Autodesk Inventor part; units mm, degrees
ref_plane "YZ Plane" through (0, 0, 0) normal (1, 0, 0) x (0, 1, 0)
ref_plane "XZ Plane" through (0, 0, 0) normal (0, 1, 0) x (-1, 0, 0)
ref_plane "XY Plane" through (0, 0, 0) normal (0, 0, 1) x (1, 0, 0)
sketch "Sketch1" plane through (0, 0, 0) normal (0, 1, 0) x (-1, 0, 0)
  line L0 (4.9, 2.9) -> (-4.9, 2.9)
  line L1 (-4.9, 2.9) -> (-4.9, -2.9)
  line L2 (-4.9, -2.9) -> (4.9, -2.9)
  line L3 (4.9, -2.9) -> (4.9, 2.9)
  point P0 (0, 0)
  dimension "d0" = 9.8
  dimension "d1" = 5.8
  dimension "d2" = 2.9
  dimension "d3" = 4.9
extrude "Extrusion1" add sketch "Sketch1" along normal blind 20
sketch "Sketch2" plane through (0, 0, 0) normal (0, -1, 0) x (1, 0, 0)
  circle A0 centre (0, 0) radius 10
  dimension "d6" = 20
extrude "Extrusion2" add sketch "Sketch2" along normal blind 3
sketch "Sketch3" plane through (0, 20, 0) normal (0, 1, 0) x (1, 0, 0)
  line L0 (-4.9, 2.9) -> (-4.9, -2.9)
  line L1 (-4.9, -2.9) -> (4.9, -2.9)
  line L2 (-4.9, 2.9) -> (4.9, 2.9)
  line L3 (4.9, 2.9) -> (4.9, -2.9)
  line L4 (4.9, -2.9) -> (-4.9, -2.9)
  line L5 (-4.9, -2.9) -> (-4.9, 2.9)
  point P0 (0, 0)
extrude "Extrusion3" cut sketch "Sketch3" against normal up to surface (20 mm away)
sketch "Sketch4" plane through (0, 0, 0) normal (1, 0, 0) x (0, 1, 0)
  circle A0 centre (9, 0) radius 10
  line L0 (-3, 10) -> (-3, -10)
  point P0 (0, 0)
  point P1 (-3, 0)
  dimension "d11" = 20
  dimension "d12" = 12
  dimension "d13" = 0
extrude "Extrusion4" cut sketch "Sketch4" along normal through all both and the other way through all
sketch "Sketch5" plane through (0, -3, 0) normal (0, -1, 0) x (1, 0, 0)
  line L0 (-4.8, 2.8) -> (4.8, 2.8)
  line L1 (4.8, 2.8) -> (4.8, -2.8)
  line L2 (4.8, -2.8) -> (-4.8, -2.8)
  line L3 (-4.8, -2.8) -> (-4.8, 2.8)
  point P0 (0, 0)
  dimension "d16" = 9.6
  dimension "d17" = 5.6
  dimension "d18" = 2.8
  dimension "d19" = 4.8
extrude "Extrusion5" add sketch "Sketch5" against normal blind 23
sketch "Sketch6" plane through (0, -3, 0) normal (0, -1, 0) x (1, 0, 0)
  line L0 (8, 10) -> (10, 10)
  line L1 (10, 10) -> (10, -10)
  line L2 (10, -10) -> (8, -10)
  line L3 (8, -10) -> (8, 10)
  line L4 (-10, 10) -> (-8, 10)
  line L5 (-8, 10) -> (-8, -10)
  line L6 (-8, -10) -> (-10, -10)
  line L7 (-10, -10) -> (-10, 10)
  circle A0 centre (0, 0) radius 10
  point P0 (-9, -10)
  point P1 (-9, 10)
  dimension "d22" = 20
  dimension "d23" = 10
  dimension "d24" = 2
  dimension "d25" = 10
  dimension "d26" = 8
  dimension "d27" = 2
  dimension "d28" = 0
  dimension "d29" = 0
extrude "Extrusion6" cut sketch "Sketch6" against normal through all contours L0 L1 A0 L3 | A0 L3 | L1 L2 L3 A0 | A0 L7 L4 L5 | L5 A0 | L5 L6 L7 A0
properties part number "Pin"
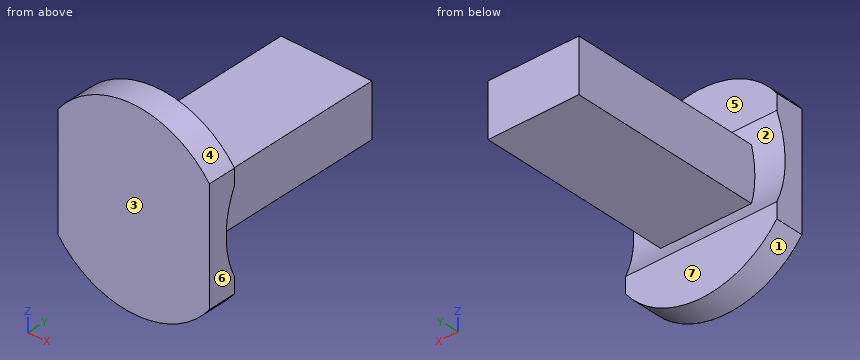
Geometry: final body of the model. Coordinates: model frame, mm. Face numbers are marked on the shaded views. A direction names the side the tool comes from. Give positions to 0.01 mm unless a question says otherwise; leave off trailing zeros. Loops run counter-clockwise (first coordinate to the right, second up) from the corner with the lowest first, then second, coordinate; pieces in that order, holes last. Notation, with made-up numbers: (-28, -18.5) -> (28, -18.5) arc R21 cw to (28, 20.5) -> close; hole circle Ø11 at (72, 58). An arc over 180 degrees is marked (long way). Use CSV: the item, a comma, the result in double quotes.
(1) Cut plane D-D (x = -2.75). Output: boundary loops of the cut face in (y, z).
From the geometry:
outline,"(-3, -9.61) -> (0, -9.61) -> (0, -4.36) arc R10 cw to (-0.6, -2.8) -> (20, -2.8) -> (20, 2.8) -> (-0.6, 2.8) arc R10 cw to (0, 4.36) -> (0, 9.61) -> (-3, 9.61) -> close"
(2) Ray query, line 1 along X through (y, z) = (0, 2.75); line 2 along Y through (x, z) = (4.5, -7.5); line 3 along Z through (x, y) = (3, 10.5). Return the intervals inside material, ascending. Write a range as [from, to].
From the geometry:
line 1,"[-4.8, 4.8]"
line 2,"[-3, 0]"
line 3,"[-2.8, 2.8]"
(3) First-contact query: P1, Ø4.5, axis at y = 11.5, z = -1, coming from the -X side; P2, Ø1.7, axis at x = 2.5, z = 6.5, coming from the +Y side; P3, Ø7.5, axis at x = 0, y = 8.5, coming from the +Z side; P4, Ø10, axis at y = 0, z = -3.5, coming from the -X side. Flat tips, straight axial feed; report the tip coordinate or a pass-through.
From the geometry:
P1,"x = -4.8"
P2,"y = 0"
P3,"z = 2.8"
P4,"x = -8"
(4) Cut plane A-A (x = 6). Output: boundary loops of the cut face in (y, z), plus the area to 3 significant figures.
From the geometry:
outline,"(-3, -8) -> (0, -8) -> (0, -4.36) arc R10 cw to (0, 4.36) -> (0, 8) -> (-3, 8) -> close"
area,"42.1 mm^2"
(5) Pull-direction query (Z, two-part tool) for the marked faces 1, 2, 3 and 4; classes: released by +Z, released by -Z, zero draft, split by the parting line, or undercut.
From the geometry:
face 1,"released by -Z"
face 2,"undercut"
face 3,"zero draft"
face 4,"released by +Z"
(6) Access query for the marked faces 5, 6 and 7. Directions: +Z, -Z, +X, -X, +Y, -Y. A direction counts if a zero-diameter tool reaches every point of the face in a straight line with its end or side. Return the directions, or none.
From the geometry:
face 5,"+Z, +X, -X, +Y"
face 6,"+Z, -Z, +X, +Y, -Y"
face 7,"-Z, +X, -X, +Y"
(7) Cut plane B-B (y = 3.5). Output: boundary loops of the cut face in (x, z), plus the area to 3 significant figures.
From the geometry:
outline,"(-4.8, -2.8) -> (4.8, -2.8) -> (4.8, 2.8) -> (-4.8, 2.8) -> close"
area,"53.8 mm^2"
(8) Cut plane C-C (z = -1). Output: boundary loops of the cut face in (x, y), plus the area to 3 significant figures.
From the geometry:
outline,"(-8, -3) -> (8, -3) -> (8, -0.95) -> (4.8, -0.95) -> (4.8, 20) -> (-4.8, 20) -> (-4.8, -0.95) -> (-8, -0.95) -> close"
area,"234 mm^2"
